```python
from build123d import *

# Parameters (mm, degrees)
SKETCH001_R     = 2.15
POCKET_DEPTH    = 3.119566
CHAMFER_SIZE    = 0.25
CHAMFER001_SIZE = 0.2


with BuildPart() as pocket:
    # Sketch003 → Revolution001 (revolve)
    with BuildSketch(Plane.XZ):
        Polygon((0, -2.118566), (1.15, -1.7), (1.15, 1), (0, 1), align=None)
    revolve(axis=Axis((0, 0, 0), (0, 0, 1)))

    # Sketch001 → Pocket (cut, through all)
    with BuildSketch(Plane(origin=(0, 0, 1), x_dir=(-1, 0, 0), z_dir=(0, 0, 1))):
        Circle(SKETCH001_R)
        Polygon((-0.57735, 1), (0.57735, 1), (1.154701, 0), (0.57735, -1), (-0.57735, -1), (-1.154701, 0), align=None, mode=Mode.SUBTRACT)
    extrude(amount=-POCKET_DEPTH, mode=Mode.SUBTRACT)


with BuildPart() as chamfer001:
    # Sketch → Revolution (revolve)
    with BuildSketch(Plane.XZ):
        Polygon((1.15, 0), (3.199999, 0), (1.5, -1.7), (1.5, -10), (0, -10), (0, -1.150001), align=None)
    revolve(axis=Axis((0, 0, 0), (0, 0, 1)))

    # Cut: cut Pocket
    add(pocket.part, mode=Mode.SUBTRACT)

    # Chamfer
    chamfer_edges = [chamfer001.edges().sort_by_distance(p)[0] for p in [
        (-3.199999, 0, 0),
    ]]
    chamfer(chamfer_edges, length=CHAMFER_SIZE)

    # Chamfer001
    chamfer001_edges = [chamfer001.edges().sort_by_distance(p)[0] for p in [
        (-1.5, 0, -10),
    ]]
    chamfer(chamfer001_edges, length=CHAMFER001_SIZE)


solid = chamfer001.part
```
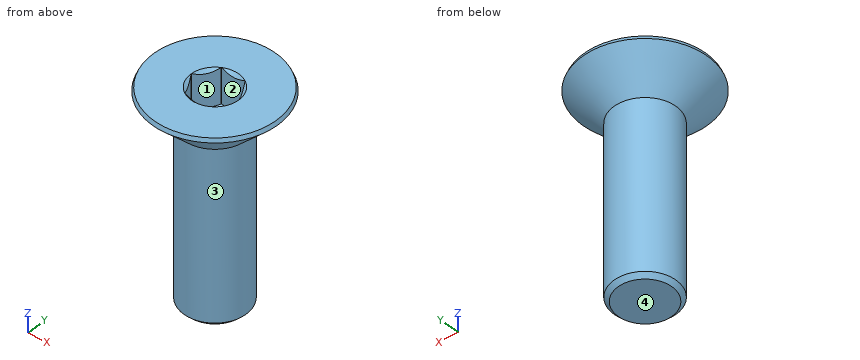
Model file for the job. Use its own axes, mm. Face numbers are marked on the shaded views. Coordinates: 2 decimals unless noted, no trailing zeros. Loops run counter-clockwise (first coordinate to the right, second up) from the corner with the lowest first, then second, coordinate; pieces in that order, holes last. Notation, with made-up numbers: (-19.75, 50.25) - (-2.75, 50.25) arc R30 ccw to (-2.75, 75.25) - close; hole circle Ø8 at (2.25, 82). An arc over 180 degrees is marked (long way). Answer as a JSON object with one key per item and string values. Group by question number.
(1) Flat gauge pins, fed straight in: pin 1 (1.2 mm diameter, centred on x = 0, z = -1, fed in from +Y); pin 2 (0.9 mm diameter, centred on x = 0, z = -1, fed in from -Y); pin 3 (2 mm diameter, centred on x = 2, z = -8, fed in from +Y). Where does each tip first touch, or does it go through?
(2) Two-plate mould, pull along Y, no slides. Class the marked faces 1, 2, 3 and 4: released by +Y, released by -Y, zero draft, split by the parting line, or undercut.
(3) Probe line 1 along Y through (x, z) = (-0.75, -5.25); line 2 along X through (y, z) = (0.5, -1); line 3 along X through (y, z) = (0.75, -0.75). List the from-to ranges inside material, lowest first.
(4) Cut at A-A (z = -2.5). Give the cut face in (x, y), then the cut area to 3 significant figures.
Geometry says:
{
 "1": {"pin 1": "stops at y = 2.8", "pin 2": "stops at y = -2.65", "pin 3": "stops at y = 1.12"},
 "2": {"face 1": "undercut", "face 2": "undercut", "face 3": "split by the parting line", "face 4": "zero draft"},
 "3": {"line 1": "y = -1.3 to 1.3", "line 2": "x = -2.14 to -0.87, 0.87 to 2.14", "line 3": "x = -2.33 to -0.72, 0.72 to 2.33"},
 "4": {"outline": "circle Ø3 at (0, 0)", "area": "7.07 mm^2"}
}
